from build123d import *

# Parameters (mm, degrees)
SKETCH4_R           = 2.375
SKETCH4_R_2         = 14
SKETCH4_R_3         = 1.5
BOSS_EXTRUDE1_DEPTH = 5
FILLET1_R           = 4
FILLET2_R           = 3
FILLET3_R           = 20
FILLET4_R           = 3


with BuildPart() as part:
    # Sketch4 → Boss-Extrude1 (new body)
    with BuildSketch(Plane.XY):
        with BuildLine():
            Line((-22.898882881, 5.245209669), (-20.836749357, -14.070107669))
            Line((-20.836749357, -14.070107669), (-0.276312074, -18.058688738))
            Line((-0.276312074, -18.058688738), (20.333519642, -14.070107669))
            Line((20.333519642, -14.070107669), (22.874540819, 5.245209669))
            Line((22.874540819, 5.245209669), (15.890720179, 5.245209669))
            ThreePointArc((15.890720179, 5.245209669), (11.856045842, 11.501579149), (5.56, 15.474054805))
            Line((5.56, 15.474054805), (5.56, 28.613702828))
            Line((5.56, 28.613702828), (0, 28.613702828))
            Line((0, 28.613702828), (-9.44, 28.613702828))
            Line((-9.44, 28.613702828), (-9.44, 19.87109493))
            Line((-9.44, 19.87109493), (-13.915384187, 19.87109493))
            Line((-13.915384187, 19.87109493), (-13.915384187, 9.41227742))
            ThreePointArc((-13.915384187, 9.41227742), (-15.200754202, 7.408655363), (-16.193820238, 5.245209669))
            Line((-16.193820238, 5.245209669), (-22.898882881, 5.245209669))
        make_face()
        with Locations((-17.729765035, -1.352900319)):
            Circle(SKETCH4_R, mode=Mode.SUBTRACT)
        with Locations((0, 17.113702828)):
            Circle(SKETCH4_R, mode=Mode.SUBTRACT)
        with Locations((17.470234965, -0.205387514)):
            Circle(SKETCH4_R, mode=Mode.SUBTRACT)
        with Locations((-0.276312074, -0.751612004)):
            Circle(SKETCH4_R_2, mode=Mode.SUBTRACT)
        with Locations((-6.44, 26.113702828)):
            Circle(SKETCH4_R_3, mode=Mode.SUBTRACT)
        with Locations((2.56, 26.113702828)):
            Circle(SKETCH4_R_3, mode=Mode.SUBTRACT)
    extrude(amount=BOSS_EXTRUDE1_DEPTH)

    # Fillet1
    fillet1_edges = [part.edges().sort_by_distance(p)[0] for p in [
        (-22.898882881, 5.245209669, 2.5),
        (22.874540819, 5.245209669, 2.5),
    ]]
    fillet(fillet1_edges, radius=FILLET1_R)

    # Fillet2
    fillet2_edges = [part.edges().sort_by_distance(p)[0] for p in [
        (-20.836749357, -14.070107669, 2.5),
        (20.333519642, -14.070107669, 2.5),
    ]]
    fillet(fillet2_edges, radius=FILLET2_R)

    # Fillet3
    fillet3_edges = [part.edges().sort_by_distance(p)[0] for p in [
        (-0.276312074, -18.058688738, 2.5),
    ]]
    fillet(fillet3_edges, radius=FILLET3_R)

    # Fillet4
    fillet4_edges = [part.edges().sort_by_distance(p)[0] for p in [
        (-13.915384187, 19.87109493, 2.5),
    ]]
    fillet(fillet4_edges, radius=FILLET4_R)


solid = part.part
Work out the finished part from the listing and answer in its coordinate system (mm). A direction names the side the tool comes from. Coordinates: 2 decimals unless noted, no trailing zeros. Order: outer loops, then holes, each group sorted by start corner. A loop starts at its lowest first (then second) coordinate and runs counter-clockwise, first axis right, second up. Notation, with made-up numbers: (-5, 72) - (32, 72) arc R8 cw to (32, 77) - close; hole circle Ø2 at (-14.5, 18). An arc over 180 degrees is marked (long way). Put each result on its own line as item: value. Start each with the question number.
1) For faces 5 (the flat face through (17, 5.245, 2)), 6 (the flat face through (-17, 5.245, 2)), 7 (the cylindrical face through (-0.33, -17.687, 2.535)), determine the directions among +Z, -Z, +X, -X, +Y, -Y from which every point of the face is accessible in a straight line to the end or side of a thin tool.
2) For a pull along X with two mould halves and no side action, classify faces 1 (the cylindrical face through (12.656, -6.114, 2.465)), 2 (the cylindrical face through (-15.185, 7.438, 2.465)), 3 (the flat face through (-10, 11, 5)), 4 (the cylindrical face through (19.81, -13.61, 2.54)) as released by +X, released by -X, zero draft, split by the parting line, or undercut.
3) Find the intervals of material crossed by line 1 (Y direction, x = -6.44, z = 2.55); line 2 (Y direction, x = 0.5, z = 1.8); line 3 (X direction, y = -3.5, z = 0.3), in increasing order. Write a range as from..to.
4) Find section A-A (y = 12.5). Give the vertices of the cut face in (x, z).
5) Find section C-C (x = 0). Give the vertices of the cut face in (y, z), plus the area to 3 significant figures.
6) Flat-ended cylindrical pins translate along their axes: pin 1 (0.7 mm diameter, centred on x = -10, z = 1.5, fed in from +Y); pin 2 (1 mm diameter, centred on y = 13.5, z = 3, fed in from -X); pin 3 (1.8 mm diameter, centred on x = -17.5, z = 2, fed in from +Y); pin 4 (5.5 mm diameter, centred on x = 0, y = 17.11, fed in from +Z). Find the tip coordinate at first contact, or state that the pin passes through.
7) Find section D-D (z = 1.3). State how many separate pieces and enclosed holes the cut face has, plus the area to 3 significant figures.
8) Find section B-B (x = 7.5). Give the vertices of the cut face in (y, z), plus the area to 3 significant figures.
Results list:
1. face 5: +Z, -Z, +X, +Y
1. face 6: +Z, -Z, -X, +Y
1. face 7: +Z, -Z, -Y
2. face 1: undercut
2. face 2: released by -X
2. face 3: zero draft
2. face 4: released by +X
3. line 1: y = -16.86..-13.32, 11.82..24.61, 27.61..28.61
3. line 2: y = -17.67..-14.73, 13.23..14.79, 19.44..28.61
3. line 3: x = -21.97..-18.74, -16.71..-14, 13.45..21.72
4. outline: (-13.92, 0) - (-4.79, 0) - (-4.79, 5) - (-13.92, 5) - close; (4.24, 0) - (10.76, 0) - (10.76, 5) - (4.24, 5) - close
5. outline: (-17.68, 0) - (-14.75, 0) - (-14.75, 5) - (-17.68, 5) - close; (13.25, 0) - (14.74, 0) - (14.74, 5) - (13.25, 5) - close; (19.49, 0) - (28.61, 0) - (28.61, 5) - (19.49, 5) - close
5. area: 67.8 mm^2
6. pin 1: stops at y = 19.87
6. pin 2: stops at x = -13.92
6. pin 3: stops at y = 5.25
6. pin 4: stops at z = 5
7. separate pieces: 1
7. enclosed holes: 6
7. area: 715 mm^2
8. outline: (-16.55, 0) - (-12.39, 0) - (-12.39, 5) - (-16.55, 5) - close; (10.89, 0) - (14.64, 0) - (14.64, 5) - (10.89, 5) - close
8. area: 39.5 mm^2
